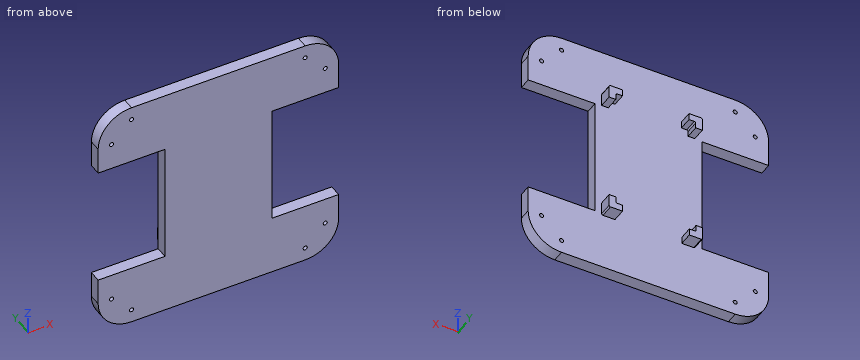
from build123d import *

# Parameters (mm, degrees)
PLATE_DEPTH               = 9
SKETCH3_R                 = 1.525
HEX_HOLES_DEPTH           = 128.597021909
RASPBERRY_PI_HOLDER_DEPTH = 10
FILLET1_R                 = 1
SKETCH5_W                 = 50
SKETCH5_H                 = 90
CUT_EXTRUDE1_DEPTH        = 128.671453348


with BuildPart() as part:
    # Sketch1 → Plate (new body)
    with BuildSketch(Plane(origin=(0, 0, 0), x_dir=(1, 0, 0), z_dir=(0, 1, 0))):
        with BuildLine():
            Line((-65, -90), (65, -90))
            ThreePointArc((65, -90), (82.67766953, -82.67766953), (90, -65))
            Line((90, -65), (90, 65))
            ThreePointArc((90, 65), (82.67766953, 82.67766953), (65, 90))
            Line((65, 90), (-65, 90))
            ThreePointArc((-65, 90), (-82.67766953, 82.67766953), (-90, 65))
            Line((-90, 65), (-90, -65))
            ThreePointArc((-90, -65), (-82.67766953, -82.67766953), (-65, -90))
        make_face()
    extrude(amount=PLATE_DEPTH)

    # Sketch3 → Hex Holes (cut, through all)
    with BuildSketch(Plane(origin=(0, 9, 0), x_dir=(1, 0, 0), z_dir=(0, 1, 0))):
        with Locations(Location((-65, 80, 0), (0, 0, 270))):
            Circle(SKETCH3_R)
        with Locations(Location((-80, 65, 0), (0, 0, 270))):
            Circle(SKETCH3_R)
        with Locations(Location((80, 65, 0), (0, 0, 270))):
            Circle(SKETCH3_R)
        with Locations(Location((80, -65, 0), (0, 0, 270))):
            Circle(SKETCH3_R)
        with Locations(Location((65, 80, 0), (0, 0, 270))):
            Circle(SKETCH3_R)
        with Locations(Location((65, -80, 0), (0, 0, 270))):
            Circle(SKETCH3_R)
        with Locations(Location((-65, -80, 0), (0, 0, 270))):
            Circle(SKETCH3_R)
        with Locations(Location((-80, -65, 0), (0, 0, 270))):
            Circle(SKETCH3_R)
    extrude(amount=-HEX_HOLES_DEPTH, mode=Mode.SUBTRACT)

    # Sketch4 → Raspberry Pi Holder (add)
    with BuildSketch(Plane(origin=(0, 9, 0), x_dir=(1, 0, 0), z_dir=(0, 1, 0))):
        Polygon((-30, 36.5), (-30, 41.5), (-25, 41.5), (-25, 46.5), (-35, 46.5), (-35, 36.5), align=None)
        Polygon((25, 46.5), (35, 46.5), (35, 36.5), (30, 36.5), (30, 41.5), (25, 41.5), align=None)
        Polygon((-34.75, -45.5), (-34.75, -55.5), (-24.75, -55.5), (-24.75, -50.5), (-29.75, -50.5), (-29.75, -45.5), align=None)
        Polygon((25, -50.5), (25, -55.5), (35, -55.5), (35, -45.5), (30, -45.5), (30, -50.5), align=None)
    extrude(amount=RASPBERRY_PI_HOLDER_DEPTH)

    # Fillet1
    fillet1_edges = [part.edges().sort_by_distance(p)[0] for p in [
        (-30, 14, -41.5),
        (-35, 14, -46.5),
        (30, 14, -41.5),
        (35, 14, -46.5),
        (-34.75, 14, 55.5),
        (-29.75, 14, 50.5),
        (35, 14, 55.5),
        (30, 14, 50.5),
    ]]
    fillet(fillet1_edges, radius=FILLET1_R)

    # Sketch5 → Cut-Extrude1 (cut, through all)
    with BuildSketch(Plane(origin=(0, 9, 0), x_dir=(1, 0, 0), z_dir=(0, 1, 0))):
        with Locations((-65, 0)):
            Rectangle(SKETCH5_W, SKETCH5_H)
        with Locations((65, 0)):
            Rectangle(SKETCH5_W, SKETCH5_H)
    extrude(amount=-CUT_EXTRUDE1_DEPTH, mode=Mode.SUBTRACT)


solid = part.part
For this review, take the finished solid that the model builds, in its own axes (mm). Give positions to 0.01 mm unless a question says otherwise; leave off trailing zeros. Loops run counter-clockwise (first coordinate to the right, second up) from the corner with the lowest first, then second, coordinate; pieces in that order, holes last. Notation, with made-up numbers: (67.25, 88.25) - (80.25, 88.25) arc R18 cw to (80.25, 106.25) - close; hole circle Ø4 at (-4, 58). An arc over 180 degrees is marked (long way). Write each question's results on one line, items separated by ' | '.
(1) For line 1 along X through (y, z) = (5.25, 65) (3 decimals); line 2 along X through (y, z) = (17.75, -43); line 3 along Z through (x, y) = (65, 5.5) (3 decimals), list the stretches that pass through material, from the lowest coordinate up.
Conclusion:
line 1: -90 to -81.525, -78.475 to 78.475, 81.525 to 90 | line 2: -35 to -25, 25 to 35 | line 3: -90 to -81.525, -78.475 to -45, 45 to 78.475, 81.525 to 90
(2) Take a section at D-D (z = 60). Give the boundary of the cut face in (x, y).
Conclusion:
outline: (-90, 0) - (90, 0) - (90, 9) - (-90, 9) - close
(3) For pin 1 Ø3 at (x, y) = (-27.5, 13) entering from +Z; pin 2 Ø5.5 at (y, z) = (16, -45) entering from -X; pin 3 Ø10 at (x, y) = (27.5, 16.5) entering from -Z, all flat-tipped, find the tip position at first contact; note any pin that passes through.
Conclusion:
pin 1: z = 55.5 | pin 2: x = -35 | pin 3: z = -46.5
(4) Take a section at C-C (z = 40.5). Give the boundary of the cut face in (x, y), then the cut area to 3 significant figures.
Conclusion:
outline: (-40, 0) - (40, 0) - (40, 9) - (-40, 9) - close | area: 720 mm^2
(5) Take a section at A-A (y = 12.25). State how many separate pieces and enclosed holes the cut face has, then the cut area to 3 significant figures.
Conclusion:
separate pieces: 4 | enclosed holes: 0 | area: 300 mm^2
